from build123d import *

# Parameters (mm, degrees)
SKETCH1_R           = 1.75
BOSS_EXTRUDE1_DEPTH = 5


with BuildPart() as part:
    # Sketch1 → Boss-Extrude1 (new body)
    with BuildSketch(Plane.XY):
        with BuildLine():
            Line((3.927550053, -314), (1.927551127, -314))
            Line((1.927551127, -314), (-13.309839226, -314))
            Line((-13.309839226, -314), (-15.309839226, -314))
            Line((-15.309839226, -314), (-15.309839226, -106.128211153))
            Line((-15.309839226, -106.128211153), (-15.309839226, -93.5))
            ThreePointArc((-15.309839226, -93.5), (-14.724052788, -92.085786438), (-13.309839226, -91.5))
            Line((-13.309839226, -91.5), (1.927551127, -91.5))
            ThreePointArc((1.927551127, -91.5), (3.342497106, -92.086519234), (3.927550053, -93.502072123))
            Line((3.927550053, -93.502072123), (3.919263706, -101.5))
            add(Edge.make_bspline(
                [(3.919263706, -101.5), (4.762029824, -124.978966699), (28.065591749, -126.82575045)],
                knots=[0, 0, 0, 1, 1, 1], degree=2))
            Line((28.065591749, -126.82575045), (43.809757496, -126.863648017))
            Line((43.809757496, -126.863648017), (43.809757496, -293.264563137))
            Line((43.809757496, -293.264563137), (28.065591749, -293.302460704))
            add(Edge.make_bspline(
                [(3.927550053, -314), (-1.943550438, -290.062596381), (28.065591749, -293.302460704)],
                knots=[0, 0, 0, 1, 1, 1], degree=2))
        make_face()
        with Locations((-11.275154001, -97.093813656)):
            Circle(SKETCH1_R, mode=Mode.SUBTRACT)
        with Locations((-1.275154001, -97.093813656)):
            Circle(SKETCH1_R, mode=Mode.SUBTRACT)
        with Locations(Location((-1.275154001, -308.406186344, 0), (0, 0, 180))):
            Circle(SKETCH1_R, mode=Mode.SUBTRACT)
        with Locations(Location((-11.275154001, -308.406186344, 0), (0, 0, 180))):
            Circle(SKETCH1_R, mode=Mode.SUBTRACT)
    extrude(amount=BOSS_EXTRUDE1_DEPTH)


solid = part.part
Could you check a few things on this model? Use its own coordinates, in mm. Give positions to 0.01 mm unless a question says otherwise; leave off trailing zeros. Order: outer loops, then holes, each group sorted by start corner. A loop starts at its lowest first (then second) coordinate and runs counter-clockwise, first axis right, second up.
1. Will this pin go through, and if not, where does the flat tip stop? P1, Ø4, axis at x = -11.28, y = -97.09, coming from the +Z side.
2. Suppose I cut it at A-A (x = 33). List the corners of the cut face in (y, z) for me.
3. We'd pull the mould along X, two halves only. Please class faces 1 (the flat face through (-15.31, -205, 2)), 2 (the cylindrical face through (-10.896, -306.698, 2.465)), 3 (the cylindrical face through (-0.896, -306.698, 2.465)), 4 (the flat face through (15, -201, 0)): pulls with the +X half, pulls with the -X half, needs draft (parallel to the pull), parting line crosses it, or undercut.
4. Suppose I cut it at B-B (z = 3.8). Give the number of separate pieces and of enclosed holes in the cut face, plus the area to 3 significant figures.
5. I need wall thicknesses on L1, parallel to Y at x = -11, z = 2.5; L2, parallel to Y at x = -12, z = 2; L3, parallel to Y at x = 31, z = 1.3. Which ranges of each line are inside material? Lowest first, please.
Solved:
1. P1: stops at z = 5
2. outline: (-293.29, 0) - (-126.84, 0) - (-126.84, 5) - (-293.29, 5) - close
3. face 1: pulls with the -X half
3. face 2: undercut
3. face 3: undercut
3. face 4: needs draft
4. separate pieces: 1
4. enclosed holes: 4
4. area: 11,000 mm2
5. L1: y = -314 to -310.13, -306.68 to -98.82, -95.37 to -91.5
5. L2: y = -314 to -310, -306.81 to -98.69, -95.5 to -91.5
5. L3: y = -293.3 to -126.83
